```python
from build123d import *

# Parameters (mm, degrees)
F0_W     = 5.5
F0_H     = 0.5
F2_SIZE  = 1
F3_R     = 1
F5_DEPTH = 6.5
F6_SIZE  = 0.3


with BuildPart() as f1:
    # F0 (on Front) → F1 (revolve)
    with BuildSketch(Plane.XZ):
        with BuildLine():
            ThreePointArc((11, 4), (5.5509008278, 2.8767272628), (0, 2.5))
            Line((0, 2.5), (0, 0))
            Line((0, 0), (5.5, 0))
            Line((5.5, 0), (11, 0))
            Line((11, 0), (11, 4))
        make_face()
        with Locations((2.75, -0.25)):
            Rectangle(F0_W, F0_H)
    revolve(axis=Axis((0, 0, 1.25), (0, 0, -1)))

    # F2
    f2_edges = [f1.edges().sort_by_distance(p)[0] for p in [
        (-11, 0, 0),
    ]]
    chamfer(f2_edges, length=F2_SIZE)

    # F3
    f3_edges = [f1.edges().sort_by_distance(p)[0] for p in [
        (-11, 0, 4),
    ]]
    fillet(f3_edges, radius=F3_R)

    # F4 (on face) → F5 (join)
    with BuildSketch(Plane(origin=(0, 0, -0.5), x_dir=(1, 0, 0), z_dir=(0, 0, -1))):
        with BuildLine():
            ThreePointArc((-0.5, 0), (-0.3535533906, 0.3535533906), (0, 0.5))
            Line((0, 0.5), (0, 4))
            ThreePointArc((0, 4), (-2.8284271247, 2.8284271247), (-4, 0))
            Line((-4, 0), (-0.5, 0))
        make_face()
        with BuildLine():
            Line((4, 0), (0.5, 0))
            ThreePointArc((0.5, 0), (0.3535533906, -0.3535533906), (0, -0.5))
            Line((0, -0.5), (0, -4))
            ThreePointArc((0, -4), (2.8284271247, -2.8284271247), (4, 0))
        make_face()
    extrude(amount=F5_DEPTH)

    # F6
    f6_edges = [f1.edges().sort_by_distance(p)[0] for p in [
        (0, -2.25, -7),
        (-2.828427, -2.828427, -7),
        (-2.25, 0, -7),
        (-0.353553, -0.353553, -7),
        (0.353553, 0.353553, -7),
        (2.25, 0, -7),
        (2.828427, 2.828427, -7),
        (0, 2.25, -7),
    ]]
    chamfer(f6_edges, length=F6_SIZE)


solid = f1.part
```
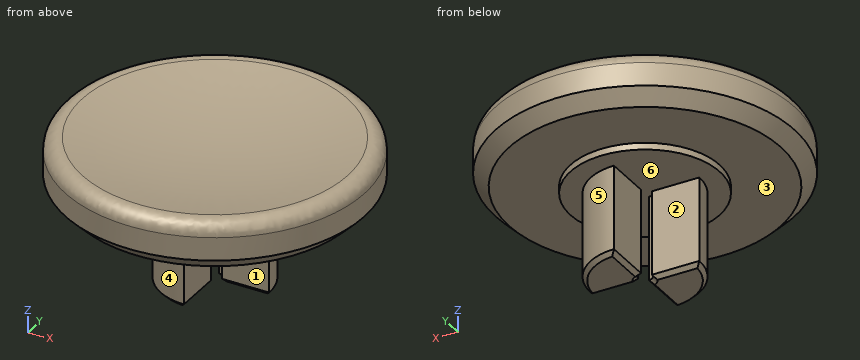
Build history of the part. All positions in model axes, mm. Face numbers are marked on the shaded views. A direction names the side the tool comes from. Round coordinates to 2 decimals unless told otherwise and drop trailing zeros. Loops run counter-clockwise (first coordinate to the right, second up) from the corner with the lowest first, then second, coordinate; pieces in that order, holes last.
Item 1: Pin check, flat tips, straight feed: P1, Ø10, axis at x = -7.5, y = -6.5, coming from the +Z side; P2, Ø5, axis at x = -6, y = -4.5, coming from the -Z side; P3, Ø1, axis at y = -1, z = -5.5, coming from the +X side; P4, Ø1.5, axis at x = 5.5, y = -7.5, coming from the -Z side. Stop position of each tip, or through.
Item 2: Saw through at B-B (z = 0.5). List the corners of the cut face in (x, y), then the cut area to 3 significant figures.
Item 3: Which spindle directions (+Z, -Z, +X, -X, +Y, -Y) get a long thin tool onto all of the face, cutting with end or side? Do the marked faces 1, 2 and 3. Say none if no direction does.
Item 4: Drill centre lines: line 1 along Z through (x, y) = (-5.25, 8.25); line 2 along Y through (x, z) = (0.25, 0.5); line 3 along X through (y, z) = (-1.5, -3). Where is each one in solid material? Low to high.
Item 5: Two-plate mould, pull along Y, no slides. Class the marked faces 4, 5 and 6: released by +Y, released by -Y, zero draft, split by the parting line, or undercut.
Item 6: Saw through at A-A (z = -2.75). List the corners of the cut face in (x, y).
Item 7: Saw through at C-C (z = 1.75). List the corners of the cut face in (x, y).
Worked answers:
1. P1: stops at z = 3.71
1. P2: stops at z = -0.5
1. P3: stops at x = 0
1. P4: stops at z = 0
2. outline: circle Ø21 at (0, 0)
2. area: 346 mm2
3. face 1: -Z, +X, -Y
3. face 2: -Z, -X, +Y
3. face 3: -Z
4. line 1: z = 0 to 3.68
4. line 2: y = -10.5 to 10.5
4. line 3: x = -3.71 to 0
5. face 4: released by -Y
5. face 5: released by +Y
5. face 6: zero draft
6. outline: (-4, 0) arc R4 ccw to (0, -4) - (0, -0.5) arc R0.5 cw to (-0.5, 0) - close; (0, 0.5) arc R0.5 cw to (0.5, 0) - (4, 0) arc R4 ccw to (0, 4) - close
7. outline: circle Ø22 at (0, 0)
